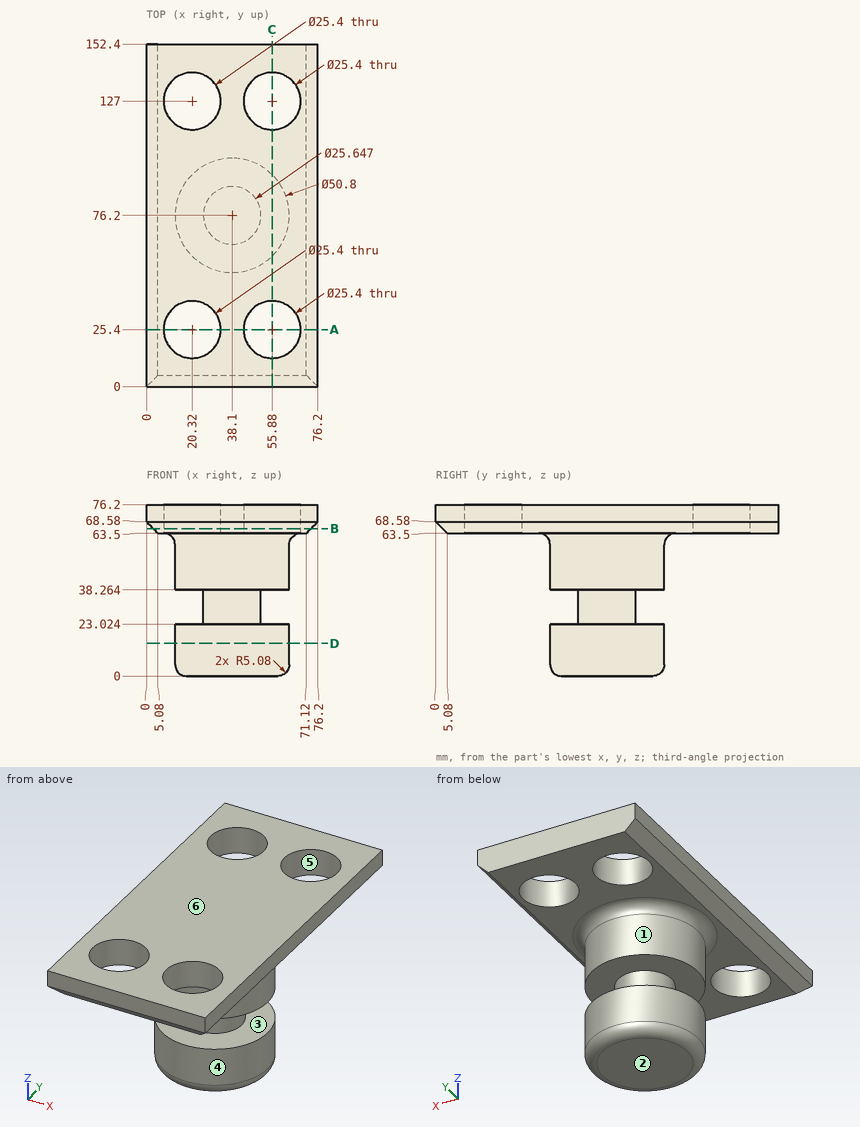
Input: dimensioned drawing with shaded views. Units: mm. Origin: part minimum x, y, z. A direction names the side the tool comes from. Coordinates: 2 decimals unless noted, no trailing zeros. Loops run counter-clockwise (first coordinate to the right, second up) from the corner with the lowest first, then second, coordinate; pieces in that order, holes last. Notation, with made-up numbers: (48.25, 61) -> (81.25, 61) arc R27 cw to (81.25, 97) -> close; hole circle Ø9 at (-11, 53.25). An arc over 180 degrees is marked (long way). One line per item, written item: value. Start each with the question number.
Q1. Section query B-B, the plane z = 65.5. Return the cut outline in (x, y).
Q2. Section query C-C, the plane x = 55.88. Give the number of separate pieces and of enclosed holes in the cut face, and give its area (3 significant figures).
Q3. Line query: line 1 along Y through (x, z) = (20.32, 72.25); line 2 along Y through (x, z) = (55.88, 68); line 3 along X through (y, z) = (130, 66.5). Output: solid intervals per line, ascending.
Q4. Mould query, pull axis X, two halves, no side actions, for the marked faces 4, 5 and 6. Classes: pulls with the +X half, pulls with the -X half, needs draft (parallel to the pull), parting line crosses it, or undercut.
Q5. Contact query for flat-ended pins moving along their axis: P1, Ø12, axis at x = 54.5, y = 94, coming from the -Z side; P2, Ø12, axis at y = 99, z = 37.5, coming from the -X side; P3, Ø10, axis at x = 34.5, y = 118.5, coming from the -Z side; P4, Ø8, axis at y = 68, z = 59, coming from the +X side. Output: stop coordinate, or through.
Q6. Section query D-D, the plane z = 14.5. Return the cut outline in (x, y).
Q7. Section query A-A, the plane y = 25.4. Return the cut outline in (x, z), and give its area (3 significant figures).
Q8. Set-up query: the marked faces 1, 2 and 3. Return all of +Z, -Z, +X, -X, +Y, -Y with unobstructed straight access to the full face (end or side cutting, diameter ignored); none if empty.
Results:
1. outline: (3.08, 3.08) -> (73.12, 3.08) -> (73.12, 152.4) -> (3.08, 152.4) -> close; hole circle Ø25.4 at (20.32, 25.4); hole circle Ø25.4 at (20.32, 127); hole circle Ø25.4 at (55.88, 25.4); hole circle Ø25.4 at (55.88, 127)
2. separate pieces: 4
2. enclosed holes: 0
2. area: 3,030 mm^2
3. line 1: 0 to 12.7, 38.1 to 114.3, 139.7 to 152.4
3. line 2: 0.58 to 12.7, 38.1 to 114.3, 139.7 to 152.4
3. line 3: 2.08 to 7.98, 32.66 to 43.54, 68.22 to 74.12
4. face 4: parting line crosses it
4. face 5: undercut
4. face 6: needs draft
5. P1: z = 0
5. P2: x = 19.09
5. P3: z = 63.5
5. P4: x = 65.25
6. outline: circle Ø50.8 at (38.1, 76.2)
7. outline: (0, 68.58) -> (5.08, 63.5) -> (7.62, 63.5) -> (7.62, 76.2) -> (0, 76.2) -> close; (33.02, 63.5) -> (43.18, 63.5) -> (43.18, 76.2) -> (33.02, 76.2) -> close; (68.58, 63.5) -> (71.12, 63.5) -> (76.2, 68.58) -> (76.2, 76.2) -> (68.58, 76.2) -> close
7. area: 297 mm^2
8. face 1: -Z
8. face 2: -Z, +X, -X, +Y, -Y
8. face 3: none
